Part print with two shaded views. Sizes in mm from the minimum x, y, z corner. Coordinates: 2 decimals unless noted, no trailing zeros. Order: outer loops, then holes, each group sorted by start corner. A loop starts at its lowest first (then second) coordinate and runs counter-clockwise, first axis right, second up.
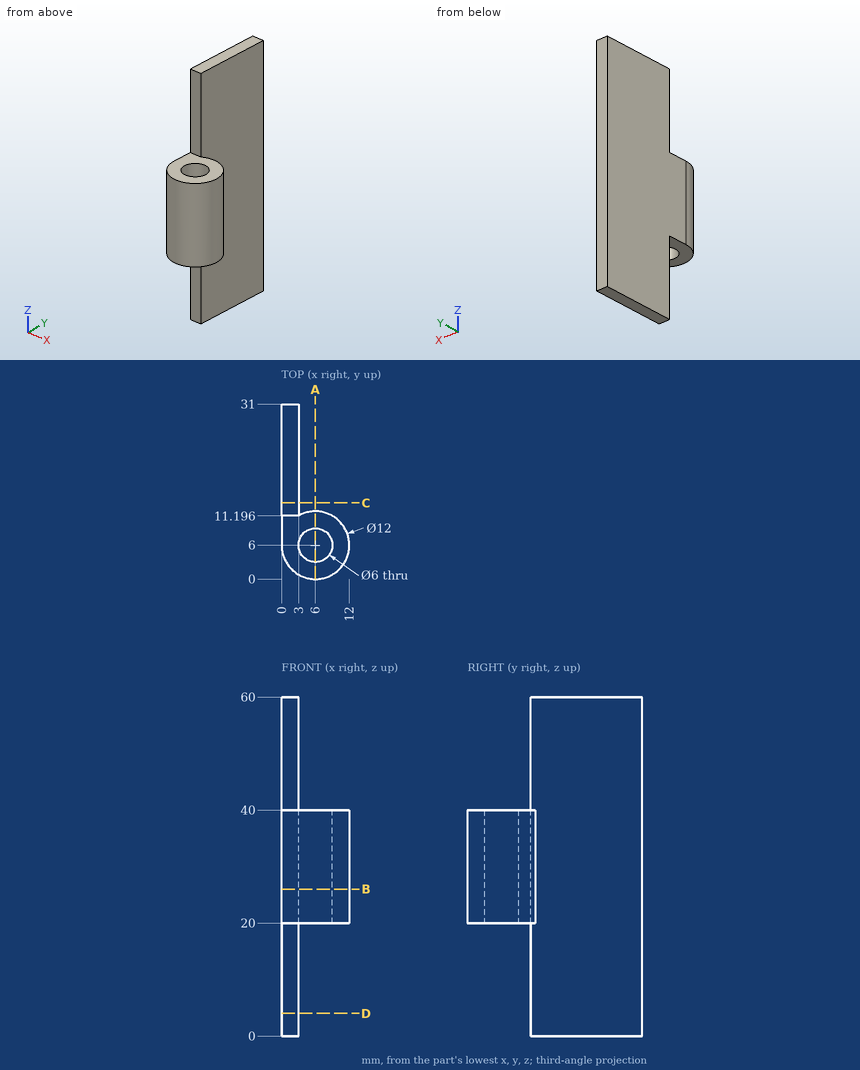
Q1. Cut at D-D on z = 4. Write the cut outline in (x, y), and give its area (3 significant figures).
Results list:
outline: (0, 11.2) - (3, 11.2) - (3, 31) - (0, 31) - close
area: 59.4 mm2
Q2. Wall check: line 1 along Y through (x, z) = (6, 27.25); line 2 along Z through (x, y) = (9.25, 5.5); line 3 along Y through (x, z) = (8, 34). Give the ranges that are in metal, low to high.
Results list:
line 1: y = 0 to 3, 9 to 12
line 2: z = 20 to 40
line 3: y = 0.34 to 3.76, 8.24 to 11.66
Q3. Cut at A-A on x = 6. Write the cut outline in (y, z).
Results list:
outline: (0, 20) - (3, 20) - (3, 40) - (0, 40) - close; (9, 20) - (12, 20) - (12, 40) - (9, 40) - close
Q4. Cut at C-C on y = 13.5. Write the cut outline in (x, z).
Results list:
outline: (0, 0) - (3, 0) - (3, 60) - (0, 60) - close
Q5. Cut at B-B on z = 26. Write the cut outline in (x, y), and give its area (3 significant figures).
Results list:
outline: (0, 6) arc R6 ccw (long way) to (3, 11.2) - (3, 31) - (0, 31) - close; hole circle Ø6 at (6, 6)
area: 149 mm2
Q6. Pin check, flat tips, straight feed: pin 1 Ø8 at (y, z) = (11, 47) entering from +X; pin 2 Ø2 at (x, z) = (8, 41.5) entering from +Y; pin 3 Ø12 at (y, z) = (15, 34.5) entering from +X; pin 4 Ø1.5 at (x, z) = (1.5, 49.5) entering from -Y. Stop position of each tip, or through.
Results list:
pin 1: stops at x = 3
pin 2: passes through
pin 3: stops at x = 11.2
pin 4: stops at y = 11.2
